Source: three-view drawing plus pictorial views. Frame: mm from the lowest corner of the part. A direction names the side the tool comes from. Round coordinates to 2 decimals unless told otherwise and drop trailing zeros. Order: outer loops, then holes, each group sorted by start corner. A loop starts at its lowest first (then second) coordinate and runs counter-clockwise, first axis right, second up. Notation, with made-up numbers: (84.25, 76.5) -> (120.25, 76.5) arc R17 cw to (120.25, 86.5) -> close; hole circle Ø9 at (-31, 21). An arc over 180 degrees is marked (long way). Answer as CSV lines item,"result". Start each with the question number.
1) Section query A-A, the plane z = 2. Output: boundary loops of the cut face in (x, y) (1 decimal).
2) Section query C-C, the plane y = 15.5. Output: boundary loops of the cut face in (x, z) (1 decimal), and give its area (3 significant figures).
3) Access query for the marked faces 1, 2 and 3. Directions: +Z, -Z, +X, -X, +Y, -Y. A direction counts if a zero-diameter tool reaches every point of the face in a straight line with its end or side. Return the directions, or none.
4) First-contact query: P1, Ø1.6, axis at x = 2, y = 13, coming from the +Z side (3 decimals); P2, Ø1, axis at x = 1.5, y = 15.5, coming from the -Z side (3 decimals). Flat tips, straight axial feed; report the tip coordinate or a pass-through.
5) Mould query, pull axis Y, two halves, no side actions, for the marked faces 4, 5 and 6. Classes: +Y half, -Y half, draft (parallel to the pull), parting line (faces both ways), or undercut.
6) Line query: L1, parallel to Y at x = 2.3, z = 17 (1 decimal); L2, parallel to Z at x = 3.05, y = 18 (1 decimal). Output: solid intervals per line, ascending.
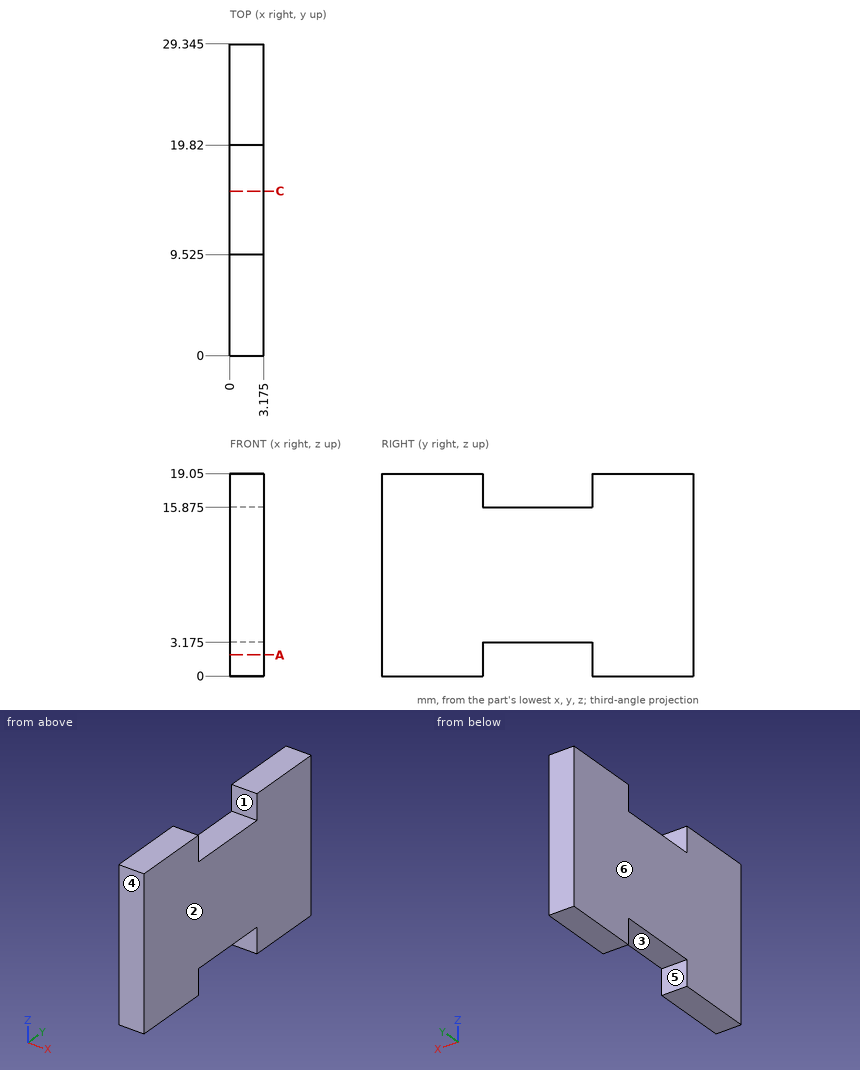
Findings:
1,outline,"(0, 0) -> (3.2, 0) -> (3.2, 9.5) -> (0, 9.5) -> close; (0, 19.8) -> (3.2, 19.8) -> (3.2, 29.3) -> (0, 29.3) -> close"
2,outline,"(0, 3.2) -> (3.2, 3.2) -> (3.2, 15.9) -> (0, 15.9) -> close"
2,area,"40.3 mm^2"
3,face 1,"+Z, +X, -X"
3,face 2,"+Z, -Z, +X, +Y, -Y"
3,face 3,"-Z, +X, -X"
4,P1,"stops at z = 15.875"
4,P2,"stops at z = 3.175"
5,face 4,"-Y half"
5,face 5,"undercut"
5,face 6,"draft"
6,L1,"y = 0 to 9.5, 19.8 to 29.3"
6,L2,"z = 3.2 to 15.9"
